The model under review builds one solid part; all positions refer to its coordinate system, in mm. Face numbers are marked on the shaded views. A direction names the side the tool comes from. Give positions to 0.01 mm unless a question says otherwise; leave off trailing zeros. Order: outer loops, then holes, each group sorted by start corner. A loop starts at its lowest first (then second) coordinate and runs counter-clockwise, first axis right, second up.
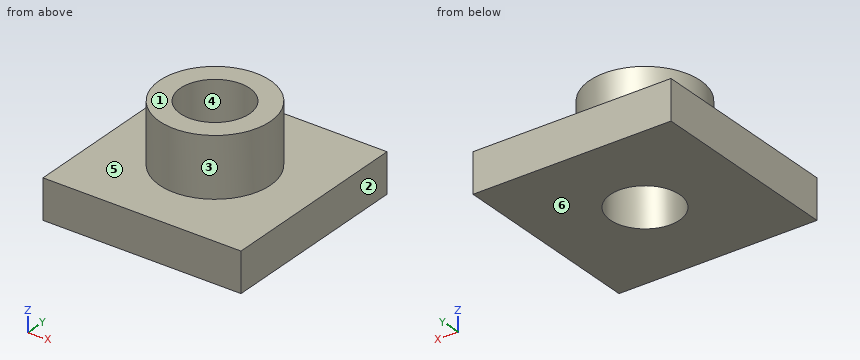
```python
from build123d import *

# Parameters (mm, degrees)
SKETCH_R        = 2.8
PAD_DEPTH       = 3
SKETCH001_R     = 1.75
POCKET_DEPTH    = 4
SKETCH002_W     = 10
SKETCH002_H     = 10
PAD001_DEPTH    = 2
SKETCH003_R     = 1.75
POCKET001_DEPTH = 5


with BuildPart() as part:
    # Sketch → Pad (new body)
    with BuildSketch(Plane.XY):
        Circle(SKETCH_R)
    extrude(amount=PAD_DEPTH)

    # Sketch001 (on Face3 of Pad) → Pocket (cut)
    with BuildSketch(Plane.XY.offset(3)):
        Circle(SKETCH001_R)
    extrude(amount=-POCKET_DEPTH, mode=Mode.SUBTRACT)

    # Sketch002 (on Face2 of Pocket) → Pad001 (join)
    with BuildSketch(Plane(origin=(0, 0, 0), x_dir=(1, 0, 0), z_dir=(0, 0, -1))):
        Rectangle(SKETCH002_W, SKETCH002_H)
    extrude(amount=PAD001_DEPTH)

    # Sketch003 (on Face10 of Pad001) → Pocket001 (cut)
    with BuildSketch(Plane.XY):
        Circle(SKETCH003_R)
    extrude(amount=-POCKET001_DEPTH, mode=Mode.SUBTRACT)


solid = part.part
```
1. Take a section at A-A (x = 0). Write out the cut boundary in (y, z).
2. Insertion check: pin 1 (1 mm diameter, centred on y = 1.5, z = 1.5, fed in from -X); pin 2 (1.5 mm diameter, centred on x = -1.5, y = -3.5, fed in from +Z); pin 3 (3 mm diameter, centred on x = 0, y = 0, fed in from +Z). Each pin has a flat end and moves straight along its axis. Give the tip position at first contact, or say it passes through.
3. To check wall thickness, follow line 1 (Y direction, x = 0, z = 0.8); line 2 (Y direction, x = 0, z = -0.85); line 3 (Z direction, x = -2, y = -3.25). State the ranges of each line that lie inside material, in increasing order.
4. For the marked faces 5 and 6, list the 3-axis set-ups (+Z, -Z, +X, -X, +Y, -Y) from which the entire face can be reached by the end or side of a thin tool; tool diameter is ignored.
5. Take a section at C-C (z = -0.85). Write out the cut boundary in (x, y), and give its area (3 significant figures).
6. Take a section at D-D (y = -3.5). Write out the cut boundary in (x, z), and give its area (3 significant figures).
7. Draft analysis for pull direction X (two halves, no side actions). For the marked faces 1, 2, 3 and 4, state which applies: pulls with the +X half, pulls with the -X half, needs draft (parallel to the pull), parting line crosses it, or undercut.
Answer:
1. outline: (-5, -2) - (-1.75, -2) - (-1.75, 3) - (-2.8, 3) - (-2.8, 0) - (-5, 0) - close; (1.75, -2) - (5, -2) - (5, 0) - (2.8, 0) - (2.8, 3) - (1.75, 3) - close
2. pin 1: stops at x = -2.62
2. pin 2: stops at z = 0
2. pin 3: passes through
3. line 1: y = -2.8 to -1.75, 1.75 to 2.8
3. line 2: y = -5 to -1.75, 1.75 to 5
3. line 3: z = -2 to 0
4. face 5: +Z
4. face 6: -Z, +X, -X, +Y, -Y
5. outline: (-5, -5) - (5, -5) - (5, 5) - (-5, 5) - close; hole circle Ø3.5 at (0, 0)
5. area: 90.4 mm2
6. outline: (-5, -2) - (5, -2) - (5, 0) - (-5, 0) - close
6. area: 20.0 mm2
7. face 1: needs draft
7. face 2: pulls with the +X half
7. face 3: parting line crosses it
7. face 4: undercut
